from build123d import *

# Parameters (mm, degrees)
EXTRUDE_400_DEPTH   = 2
FILLET_1302_R       = 0.1
SKETCH_7_R          = 3.348684761
CUT_EXTRUDE_1_DEPTH = 9


with BuildPart() as part:
    # 草图1 → Extrude 400 (new body)
    with BuildSketch(Plane(origin=(0, 0, 0), x_dir=(0, 0, -1), z_dir=(1, 0, 0))):
        Polygon((2.75, 1.58771324), (2.75, -1.58771324), (0, -3.175426481), (-2.75, -1.58771324), (-2.75, 1.58771324), (0, 3.175426481), align=None)
    extrude(amount=EXTRUDE_400_DEPTH)

    # 草图2 → 凸台-旋转1 (revolve)
    with BuildSketch(Plane.XY, mode=Mode.PRIVATE) as revolve_1_sk:
        Polygon((0, 0), (27, 0), (27, 1.067), (27, 1.5), (0, 1.5), align=None)
    revolve(revolve_1_sk.sketch.rotate(Axis((0, 0, 0), (1, 0, 0)), 90), axis=Axis((0, 0, 0), (1, 0, 0)))

    # 草图3 → 切除-旋转1 (revolve, cut)
    with BuildSketch(Plane.XY):
        Polygon((0, 2.75), (3.132371439, 8.175426481), (3.132371439, 13.175426481), (-10, 13.175426481), (-10, 2.75), align=None)
    revolve(axis=Axis((0, 0, 0), (1, 0, 0)), mode=Mode.SUBTRACT)

    # 草图4 → 切除-旋转3 (revolve, cut)
    with BuildSketch(Plane.XY, mode=Mode.PRIVATE) as cut_revolve_3_sk:
        Polygon((2, 2.285), (1.7, 2.458205081), (1.7, 3.175426481), (2, 3.175426481), align=None)
    revolve(cut_revolve_3_sk.sketch.rotate(Axis((0, 0, 0), (1, 0, 0)), 90), axis=Axis((0, 0, 0), (1, 0, 0)), mode=Mode.SUBTRACT)

    # Fillet 1302
    fillet_1302_edges = [part.edges().sort_by_distance(p)[0] for p in [
        (2, 0, -1.5),
    ]]
    fillet(fillet_1302_edges, radius=FILLET_1302_R)

    # 草图6 → 切除-旋转4 (revolve, cut)
    with BuildSketch(Plane.XY, mode=Mode.PRIVATE) as cut_revolve_4_sk:
        Polygon((26.75, 1.5), (27.25, 1.5), (27, 1.066987298), align=None)
    revolve(cut_revolve_4_sk.sketch.rotate(Axis((0, 0, 0), (1, 0, 0)), 90), axis=Axis((0, 0, 0), (1, 0, 0)), mode=Mode.SUBTRACT)

    # 草图7 → 切除-拉伸1 (cut)
    with BuildSketch(Plane(origin=(27, 0, 0), x_dir=(0, 0, -1), z_dir=(1, 0, 0))):
        Circle(SKETCH_7_R)
    extrude(amount=-CUT_EXTRUDE_1_DEPTH, mode=Mode.SUBTRACT)


solid = part.part
CAD build for the part. Positions are in the model's coordinates, mm. A direction names the side the tool comes from. Coordinates: 2 decimals unless noted, no trailing zeros. Write each loop counter-clockwise with the first axis right and the second up, starting at its lowest first coordinate (ties: lowest second). Pieces come first, ordered by that corner, then holes. Notation, with made-up numbers: (-17.75, 24) - (39.25, 24) arc R31 ccw to (39.25, 48) - close; hole circle Ø7 at (-5, -7). An arc over 180 degrees is marked (long way). Use a Markdown table: item, result. Add a question column.
Item 1: 3-axis set-ups, long thin cutter, end or side, ignore diameter. For faces 1 (the face through (0.84, -2.39, 1.36)), 2 (the face through (2, 0, -2)): which of +Z, -Z, +X, -X, +Y, -Y reach the whole face in a straight line?
Item 2: Flat gauge pins, fed straight in: pin 1 (1.5 mm diameter, centred on x = 8.5, z = -0.5, fed in from -Y); pin 2 (3 mm diameter, centred on y = 1, z = -1.5, fed in from +X); pin 3 (1.5 mm diameter, centred on x = 7, y = 0, fed in from -Z); pin 4 (1.5 mm diameter, centred on x = 8, y = -1, fed in from +Z). Where does each tip first touch, or does it go through?
Item 3: Band-saw the part on A-A, the plane x = 14. Give the cut face in (y, z).
Item 4: Drill centre lines: L1, parallel to X at y = -0.5, z = 1.95; L2, parallel to X at y = -1.25, z = -2.25; L3, parallel to Y at x = 16.5, z = 0.05. Where is each one in solid material? Low to high. Write a range as from..to.
Numbers:
| question | item | result |
|---|---|---|
| 1 | face 1 | +Z, +X, -X, -Y |
| 1 | face 2 | +X |
| 2 | pin 1 | y = -1.5 |
| 2 | pin 2 | x = 18 |
| 2 | pin 3 | z = -1.5 |
| 2 | pin 4 | z = 1.48 |
| 3 | outline | circle Ø3 at (0, 0) |
| 4 | L1 | 0..2 |
| 4 | L2 | 0..1.7 |
| 4 | L3 | -1.5..1.5 |
